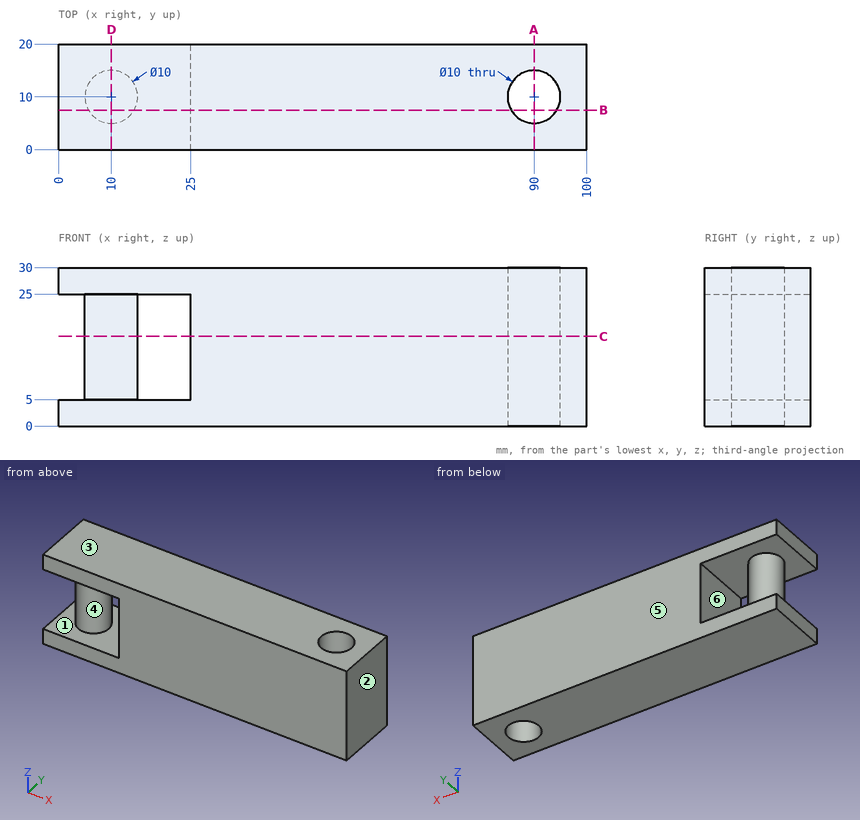
Can you work these out from the drawing? Everything is in mm from the part's minimum corner. A direction names the side the tool comes from. Give positions to 0.01 mm unless a question says otherwise; leave off trailing zeros. Order: outer loops, then holes, each group sorted by start corner. A loop starts at its lowest first (then second) coordinate and runs counter-clockwise, first axis right, second up.
Item 1: If we section it at A-A, the plane x = 90: Write out the boundary of the cut face in (y, z).
Item 2: If we mould it in two halves opening along X, with no side actions, what happens to the marked faces 1, 2 and 3? For each: pulls with the +X half, pulls with the -X half, needs draft (parallel to the pull), parting line crosses it, or undercut.
Item 3: If we section it at D-D, the plane x = 10: Write out the boundary of the cut face in (y, z), plus the area to 3 significant figures.
Item 4: For the marked faces 4, 5 and 6, which set-ups out of +Z, -Z, +X, -X, +Y, -Y let a thin tool reach every point of the face, with its end or its side?
Item 5: If we section it at C-C, the plane z = 17: Write out the boundary of the cut face in (x, y).
Item 6: If we section it at B-B, the plane y = 7.5: Write out the boundary of the cut face in (x, z), plus the area to 3 significant figures.
Item 7: I need wall thicknesses on line 1 (Z direction, x = 8, y = 3); line 2 (X direction, y = 9.5, z = 20.25); line 3 (Y direction, x = 90, z = 19.25). Which ranges of each line are inside material? Lowest first, please.
Item 8: I'm going to push flat-ended pins straight in: pin 1 (11.5 mm diameter, centred on x = 90, y = 10, fed in from -Z); pin 2 (3 mm diameter, centred on y = 14, z = 11.5, fed in from -X). Where does each tip first touch, or does it pass through?
Values:
1. outline: (0, 0) - (5, 0) - (5, 30) - (0, 30) - close; (15, 0) - (20, 0) - (20, 30) - (15, 30) - close
2. face 1: undercut
2. face 2: pulls with the +X half
2. face 3: needs draft
3. outline: (0, 0) - (20, 0) - (20, 5) - (15, 5) - (15, 25) - (20, 25) - (20, 30) - (0, 30) - (0, 25) - (5, 25) - (5, 5) - (0, 5) - close
3. area: 400 mm2
4. face 4: none
4. face 5: +Z, -Z, +X, -X, +Y
4. face 6: +Y, -Y
5. outline: circle Ø10 at (10, 10); (25, 0) - (100, 0) - (100, 20) - (25, 20) - close; hole circle Ø10 at (90, 10)
6. outline: (0, 0) - (85.67, 0) - (85.67, 30) - (0, 30) - (0, 25) - (5.67, 25) - (5.67, 5) - (0, 5) - close; (94.33, 0) - (100, 0) - (100, 30) - (94.33, 30) - close; hole (14.33, 5) - (25, 5) - (25, 25) - (14.33, 25) - close
6. area: 2,410 mm2
7. line 1: z = 0 to 5, 25 to 30
7. line 2: x = 5.03 to 14.97, 25 to 85.03, 94.97 to 100
7. line 3: y = 0 to 5, 15 to 20
8. pin 1: stops at z = 0
8. pin 2: stops at x = 5.67
